Can you work these out from the drawing? Everything is in mm from the part's minimum corner. A direction names the side the tool comes from. Round coordinates to 2 decimals unless told otherwise and drop trailing zeros. Write each loop counter-clockwise with the first axis right and the second up, starting at its lowest first coordinate (ties: lowest second). Pieces come first, ordered by that corner, then holes. Notation, with made-up numbers: (70, -10) -> (92, -10) arc R17 cw to (92, 19) -> close; hole circle Ø2 at (41.5, 11.25). An arc over 180 degrees is marked (long way). Put each result on its own line as item: value. Start each with the question number.
1. Suppose I cut it at C-C (x = 18). Please give me the cut outline in (y, z), then the cut area to 4 significant figures.
2. Which directions (+Z, -Z, +X, -X, +Y, -Y) give clear straight access to the entire face, cutting with the end or side of a thin tool? Please do the marked faces 1, 2 and 3.
3. Suppose I cut it at A-A (y = 17). Please give me the cut outline in (x, z).
4. Suppose I cut it at B-B (z = 56.5). Please give me the cut outline in (x, y), then the cut area to 3 significant figures.
5. For pin 1 (12 mm diameter, centred on x = 86.5, y = 24.5, fed in from +Z); pin 2 (20 mm diameter, centred on y = 23, z = 47, fed in from +X); pin 3 (12 mm diameter, centred on x = 66, y = 30, fed in from -Z); pin 4 (12 mm diameter, centred on y = 11.5, z = 41.5, fed in from -X), each with a flat end and sliding along its axis, tell me the tip position at first contact or that it passes through.
6. I need wall thicknesses on probe 1 along Z at (x, y) = (19, 24.5); probe 2 along X at (y, z) = (24, 36.5); probe 3 along X at (y, z) = (20.5, 32). Which ranges of each line are inside material? Lowest first, please. Write a range as from..to.
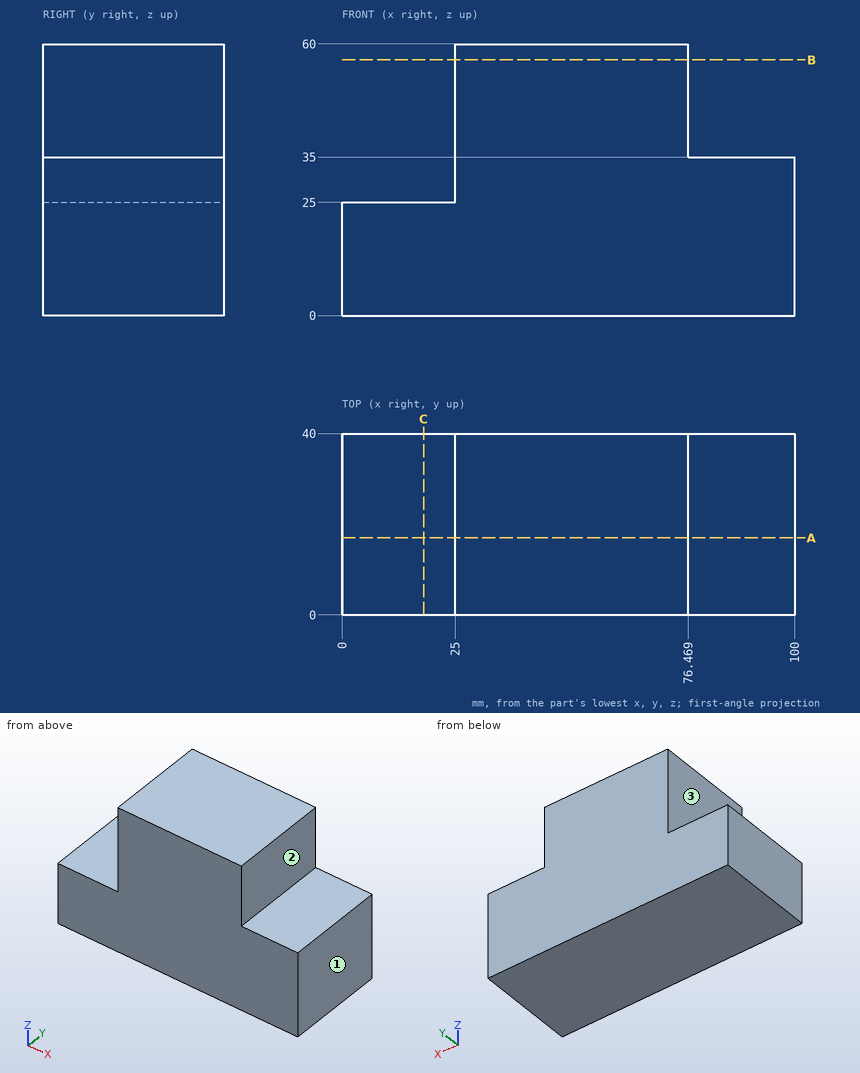
Verdict:
1. outline: (0, 0) -> (40, 0) -> (40, 25) -> (0, 25) -> close
1. area: 1,000 mm^2
2. face 1: +Z, -Z, +X, +Y, -Y
2. face 2: +Z, +X, +Y, -Y
2. face 3: +Z, -X, +Y, -Y
3. outline: (0, 0) -> (100, 0) -> (100, 35) -> (76.47, 35) -> (76.47, 60) -> (25, 60) -> (25, 25) -> (0, 25) -> close
4. outline: (25, 0) -> (76.47, 0) -> (76.47, 40) -> (25, 40) -> close
4. area: 2,060 mm^2
5. pin 1: stops at z = 35
5. pin 2: stops at x = 76.47
5. pin 3: stops at z = 0
5. pin 4: stops at x = 25
6. probe 1: z = 0..25
6. probe 2: x = 25..76.47
6. probe 3: x = 25..100
